The listing builds one solid part. Answer for the finished solid, in the listing's coordinates (mm). A direction names the side the tool comes from. Give positions to 0.01 mm unless a question says otherwise; leave off trailing zeros. Loops run counter-clockwise (first coordinate to the right, second up) from the corner with the lowest first, then second, coordinate; pieces in that order, holes last. Notation, with made-up numbers: (68, -4.5) - (89, -4.5) arc R12 cw to (89, 15.5) - close; hole circle Ø10 at (33.5, 59.5). An arc over 180 degrees is marked (long way). Write item = value, one per line. Start each with the question number.
1) Which of the six approach directions +Z, -Z, +X, -X, +Y, -Y give full straight-line access (tool end or side, diameter ignored) to faces 1 (the flat face through (44, 2, 109)), 2 (the flat face through (-45.6, 2, -111)), 3 (the flat face through (0, 2, -109)), 4 (the flat face through (61, 2, -109)), 5 (the flat face through (73, 2, -14))?
2) The part is cut by section A-A on x = 57. Write down the section's boundary in (y, z), plus the area to 3 significant figures.
3) Consider probe 1 along X at (y, z) = (1.55, -104); probe 2 along Z at (x, y) = (67, 0.4); probe 3 along X at (y, z) = (2.2, -85). Determine where each line is inside the solid, lowest interval first.
4) The part is cut by section B-B on z = 44.5. Write down the section's boundary in (x, y).
5) Flat-ended cylindrical pins translate along their axes: P1, Ø2.5, axis at x = 54, y = 2.5, coming from the +Z side; P2, Ø1.5, axis at y = 2, z = -112, coming from the -X side; P3, Ø1.5, axis at x = 74.5, y = 3.5, coming from the +Z side; P4, Ø3, axis at x = -60, z = 55.5, coming from the -Y side. Find the tip coordinate at first contact, or state that the pin passes through.
6) The mould has two halves that part along Z. Classify faces 6 (the flat face through (-76, 2, -97)), 7 (the flat face through (73, 2, 43)), 8 (the flat face through (73, 2, -71)), 9 (the flat face through (31, 2, -114)): +Z half, -Z half, draft (parallel to the pull), parting line (faces both ways), or undercut.
from build123d import *

# Parameters (mm, degrees)
BOSS_EXTRUDE1_DEPTH = 5
SKETCH2_R           = 1.6
CUT_EXTRUDE1_DEPTH  = 138.102151697
CHAMFER1_SIZE       = 1.5


with BuildPart() as part:
    # Sketch1 → Boss-Extrude1 (new body)
    with BuildSketch(Plane(origin=(0, 0, 0), x_dir=(1, 0, 0), z_dir=(0, 1, 0))):
        Polygon((0, -114), (-15.2, -114), (-15.2, -109), (-73, -109), (-73, -85.5), (-76, -85.5), (-76, -57), (-73, -57), (-73, -28.5), (-76, -28.5), (-76, 0), (-73, 0), (-73, 28.5), (-76, 28.5), (-76, 57), (-73, 57), (-73, 85.5), (-76, 85.5), (-76, 109), (-45.6, 109), (-45.6, 114), (-15.2, 114), (-15.2, 109), (0, 109), align=None)
    boss_extrude1 = extrude(amount=BOSS_EXTRUDE1_DEPTH)

    # Mirror1: Boss-Extrude1 across plane
    add(boss_extrude1.mirror(Plane(origin=(0, 5, 0), x_dir=(0, 0, 1), z_dir=(1, 0, 0))))

    # Sketch2 → Cut-Extrude1 (cut, through all)
    with BuildSketch(Plane(origin=(0, 5, 0), x_dir=(1, 0, 0), z_dir=(0, 1, 0))):
        with Locations(Location((0, 104, 0), (0, 0, 270))):
            Circle(SKETCH2_R)
    extrude(amount=-CUT_EXTRUDE1_DEPTH, mode=Mode.SUBTRACT)

    # Chamfer1
    chamfer1_edges = [part.edges().sort_by_distance(p)[0] for p in [
        (0, 5, -105.6),
    ]]
    chamfer(chamfer1_edges, length=CHAMFER1_SIZE)


solid = part.part
Answer below:
q1.face_1 = +Z, +X, +Y, -Y
q1.face_2 = -Z, -X, +Y, -Y
q1.face_3 = -Z, +Y, -Y
q1.face_4 = -Z, +X, +Y, -Y
q1.face_5 = +X, +Y, -Y
q2.outline = (0, -109) - (5, -109) - (5, 109) - (0, 109) - close
q2.area = 1,090 mm2
q3.probe_1 = -76 to -1.6, 1.6 to 76
q3.probe_2 = -109 to 109
q3.probe_3 = -73 to 73
q4.outline = (-73, 0) - (73, 0) - (73, 5) - (-73, 5) - close
q5.P1 = 109
q5.P2 = -45.6
q5.P3 = 85.5
q5.P4 = 0
q6.face_6 = draft
q6.face_7 = undercut
q6.face_8 = undercut
q6.face_9 = -Z half
